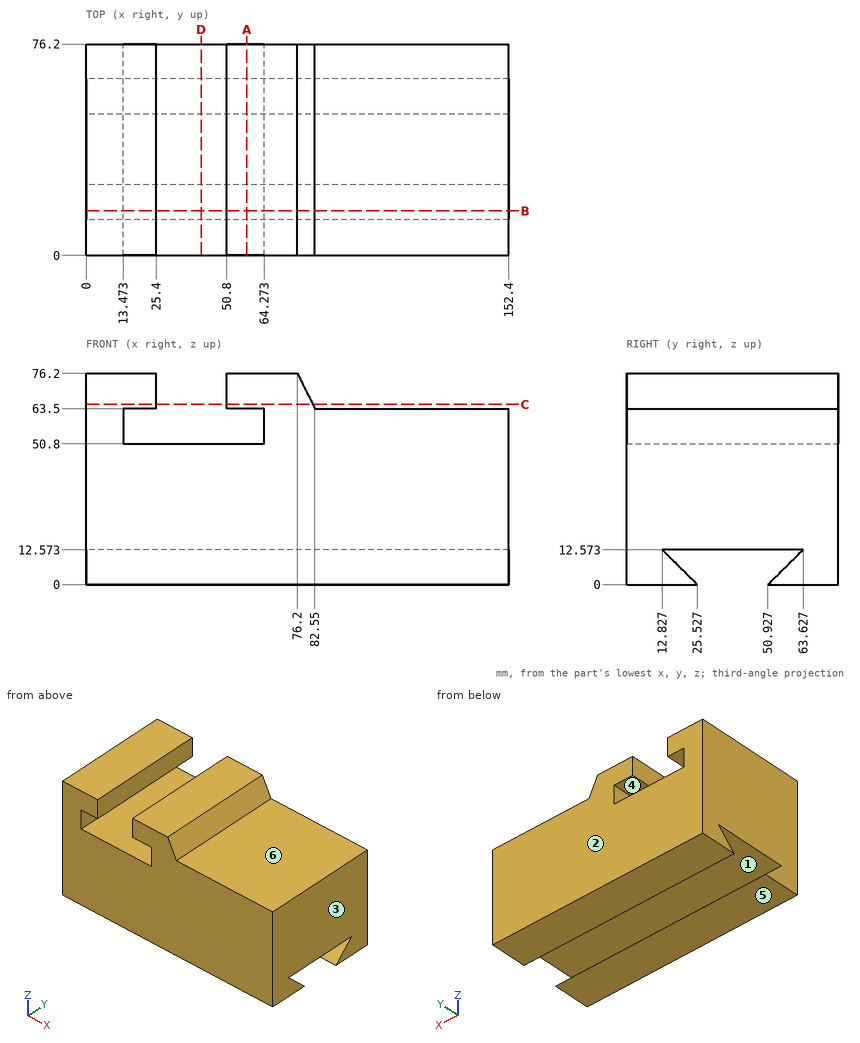
For this review, use the dimensioned drawing (mm, ordinates from the lowest corner) and the shaded views. A direction names the side the tool comes from. Coordinates: 2 decimals unless noted, no trailing zeros. Loops run counter-clockwise (first coordinate to the right, second up) from the corner with the lowest first, then second, coordinate; pieces in that order, holes last. Notation, with made-up numbers: (-11, 7) -> (29, 7) arc R13 cw to (29, 25) -> close; hole circle Ø2 at (68.5, 20.5). An arc over 180 degrees is marked (long way). Return JSON: item names as keys, results as strings. Group by question number.
(1) Consider section D-D, the plane x = 41.5. Give the boundary of the cut face in (y, z), plus the area to 3 significant figures.
(2) Tool access review of the marked faces 4, 5 and 6: name each direction out of +Z, -Z, +X, -X, +Y, -Y from which nothing blocks a thin tool from reaching the whole face with its end or side.
(3) For pin 1 Ø1 at (x, y) = (114, 38) entering from +Z; pin 2 Ø15 at (x, y) = (47.5, 33) entering from +Z; pin 3 Ø4 at (y, z) = (9.5, 66.5) entering from +X; pin 4 Ø10 at (x, y) = (106, 36) entering from -Z, all flat-tipped, find the tip position at first contact; note any pin that passes through.
(4) Consider section C-C, the plane z = 65. Give the boundary of the cut face in (x, y), plus the area to 3 significant figures.
(5) To check wall thickness, follow L1, parallel to Z at x = 24.5, y = 19.5 (1 decimal); L2, parallel to Z at x = 20, y = 41.5; L3, parallel to X at y = 63.5, z = 56. State the ranges of each line that lie inside material, in increasing order.
(6) Consider section A-A, the plane x = 58. Give the boundary of the cut face in (y, z), plus the area to 3 significant figures.
(7) Mouldability with a two-part tool opening along Y and no side actions: class the marked faces 1, 2 and 3 as pulls with the +Y half, pulls with the -Y half, needs draft (parallel to the pull), parting line crosses it, or undercut.
(8) Consider section B-B, the plane y = 16. Give the boundary of the cut face in (x, z), plus the area to 3 significant figures.
Results below:
{
 "1": {"outline": "(0, 0) -> (25.53, 0) -> (12.83, 12.57) -> (63.63, 12.57) -> (50.93, 0) -> (76.2, 0) -> (76.2, 50.8) -> (0, 50.8) -> close", "area": "3,390 mm2"},
 "2": {"face 4": "+Y, -Y", "face 5": "-Z, +X, -X, +Y, -Y", "face 6": "+Z, +X, +Y, -Y"},
 "3": {"pin 1": "stops at z = 63.5", "pin 2": "stops at z = 76.2", "pin 3": "stops at x = 82.05", "pin 4": "stops at z = 12.57"},
 "4": {"outline": "(0, 0) -> (25.4, 0) -> (25.4, 76.2) -> (0, 76.2) -> close; (50.8, 0) -> (81.8, 0) -> (81.8, 76.2) -> (50.8, 76.2) -> close", "area": "4,300 mm2"},
 "5": {"L1": "z = 0 to 6, 12.6 to 50.8, 63.5 to 76.2", "L2": "z = 12.57 to 50.8, 63.5 to 76.2", "L3": "x = 0 to 13.47, 64.27 to 152.4"},
 "6": {"outline": "(0, 0) -> (25.53, 0) -> (12.83, 12.57) -> (63.63, 12.57) -> (50.93, 0) -> (76.2, 0) -> (76.2, 50.8) -> (0, 50.8) -> close; (0, 63.5) -> (76.2, 63.5) -> (76.2, 76.2) -> (0, 76.2) -> close", "area": "4,360 mm2"},
 "7": {"face 1": "undercut", "face 2": "pulls with the +Y half", "face 3": "needs draft"},
 "8": {"outline": "(0, 0) -> (152.4, 0) -> (152.4, 9.43) -> (0, 9.43) -> close; (0, 12.57) -> (152.4, 12.57) -> (152.4, 63.5) -> (82.55, 63.5) -> (76.2, 76.2) -> (50.8, 76.2) -> (50.8, 63.5) -> (64.27, 63.5) -> (64.27, 50.8) -> (13.47, 50.8) -> (13.47, 63.5) -> (25.4, 63.5) -> (25.4, 76.2) -> (0, 76.2) -> close", "area": "9,240 mm2"}
}
